```python
from build123d import *

# Parameters (mm, degrees)
SKETCH_1_R      = 11.5
SKETCH_1_R_2    = 8.5
EXTRUDE_1_DEPTH = 4
SKETCH_2_R      = 12.25
SKETCH_2_R_2    = 11.5
EXTRUDE_2_DEPTH = 0.8
FILLET_1_R      = 0.2


with BuildPart() as part:
    # ｽｹｯﾁ1 → 押し出し-薄板1 (new body)
    with BuildSketch(Plane.XY):
        Circle(SKETCH_1_R)
        Circle(SKETCH_1_R_2, mode=Mode.SUBTRACT)
    extrude(amount=EXTRUDE_1_DEPTH)

    # ｽｹｯﾁ2 → 押し出し-薄板2 (add)
    with BuildSketch(Plane(origin=(0, 0, 0), x_dir=(-1, 0, 0), z_dir=(0, 0, -1))):
        Circle(SKETCH_2_R)
        Circle(SKETCH_2_R_2, mode=Mode.SUBTRACT)
    extrude(amount=-EXTRUDE_2_DEPTH)

    # ﾌｨﾚｯﾄ1
    fillet_1_edges = [part.edges().sort_by_distance(p)[0] for p in [
        (-8.5, 0, 0),
        (-8.5, 0, 4),
    ]]
    fillet(fillet_1_edges, radius=FILLET_1_R)


solid = part.part
```
Check sheet for the modelled part. Datum: model origin and axes. Units: mm. A direction names the side the tool comes from. Coordinates: 2 decimals unless noted, no trailing zeros. Write each loop counter-clockwise with the first axis right and the second up, starting at its lowest first coordinate (ties: lowest second). Pieces come first, ordered by that corner, then holes. Notation, with made-up numbers: (26.5, 32) - (84.5, 32) arc R31 ccw to (84.5, 70) - close; hole circle Ø5 at (-30, -36.5). An arc over 180 degrees is marked (long way). One line per question, with ' | ' between items.
Item 1: Sectioned sample at D-D on z = 2.35. Record the boundary of the cut face in (x, y).
Determined:
outline: circle Ø23 at (0, 0); hole circle Ø17 at (0, 0)
Item 2: Sectioned sample at A-A on y = 0. Record the boundary of the cut face in (x, z).
Determined:
outline: (-12.25, 0) - (-8.7, 0) arc R0.2 ccw to (-8.5, 0.2) - (-8.5, 3.8) arc R0.2 ccw to (-8.7, 4) - (-11.5, 4) - (-11.5, 0.8) - (-12.25, 0.8) - close; (8.5, 0.2) arc R0.2 ccw to (8.7, 0) - (12.25, 0) - (12.25, 0.8) - (11.5, 0.8) - (11.5, 4) - (8.7, 4) arc R0.2 ccw to (8.5, 3.8) - close
Item 3: Mould release check, pull along X, two halves, no side actions. Record for faces 3 (the face through (4.57, 7.167, 1.975)), 4 (the face through (-6.586, 10.329, 0.394)), 5 (the face through (-5, -8, 0)): pulls with the +X half, pulls with the -X half, needs draft (parallel to the pull), parting line crosses it, or undercut.
Determined:
face 3: undercut | face 4: parting line crosses it | face 5: needs draft
Item 4: Thickness scan on line 1 (Y direction, x = 0, z = 2.8); line 2 (Z direction, x = -6.25, y = -10); line 3 (Y direction, x = -2.5, z = 0.6). Record the ranges inside material, lowest first. Write a range as [from, to].
Determined:
line 1: y = [-11.5, -8.5], [8.5, 11.5] | line 2: z = [0, 0.8] | line 3: y = [-11.99, -8.12], [8.12, 11.99]
Item 5: Access from +Z, -Z, +X, -X, +Y, -Y to the whole of each face (thin tool, end or side, straight path). Record for faces 1 (the face through (11, -4, 0.8)), 2 (the face through (-2, 9, 4)).
Determined:
face 1: +Z | face 2: +Z, +X, -X, +Y, -Y
Item 6: Sectioned sample at C-C on x = 10. Record the boundary of the cut face in (y, z), plus the area to 3 significant figures.
Determined:
outline: (-7.08, 0) - (7.08, 0) - (7.08, 0.8) - (5.68, 0.8) - (5.68, 4) - (-5.68, 4) - (-5.68, 0.8) - (-7.08, 0.8) - close | area: 47.7 mm2
Item 7: Gauge pin test, flat ends, axial feed: P1, Ø1, axis at y = 3.5, z = 0.5, coming from the +X side; P2, Ø2, axis at y = -9, z = 3, coming from the +X side; P3, Ø2, axis at y = -1, z = 2, coming from the -X side. Record the tip position at first contact, or that the pin passes through.
Determined:
P1: stops at x = 11.88 | P2: stops at x = 8.26 | P3: stops at x = -11.5
